```python
from build123d import *

# Parameters (mm, degrees)
SKETCH_1_R          = 3.4
EXTRUDE_1_DEPTH     = 11
SKETCH_2_R          = 3.4
EXTRUDE_2_DEPTH     = 3
SKETCH_3_R          = 3.4
CUT_EXTRUDE_1_DEPTH = 28.083205128
CUT_EXTRUDE_START   = -5
SKETCH_4_R          = 6
SKETCH_4_R_2        = 3.4
CUT_EXTRUDE_2_DEPTH = 5
CUT_EXTRUDE_3_DEPTH = 28.083205128
CUT_EXTRUDE_5_DEPTH = 28.083205128
SKETCH_8_R          = 3.4
EXTRUDE_3_DEPTH     = 1
CUT_EXTRUDE_START_2 = -1
CUT_EXTRUDE_6_DEPTH = 1
CUT_EXTRUDE_7_DEPTH = 1
CUT_EXTRUDE_START_3 = -10
CUT_EXTRUDE_8_DEPTH = 10
EXTRUDE_START       = -4
SKETCH_12_R         = 6
SKETCH_12_R_2       = 3.25
EXTRUDE_5_DEPTH     = 4


with BuildPart() as part:
    # 草图1 → 凸台-拉伸1 (new body)
    with BuildSketch(Plane.XY):
        with BuildLine():
            Line((-9.5, -17.5), (9.5, -17.5))
            ThreePointArc((9.5, -17.5), (15.156854249, -15.156854249), (17.5, -9.5))
            Line((17.5, -9.5), (17.5, 9.5))
            ThreePointArc((17.5, 9.5), (15.156854249, 15.156854249), (9.5, 17.5))
            Line((9.5, 17.5), (-9.5, 17.5))
            ThreePointArc((-9.5, 17.5), (-15.156854249, 15.156854249), (-17.5, 9.5))
            Line((-17.5, 9.5), (-17.5, -9.5))
            ThreePointArc((-17.5, -9.5), (-15.156854249, -15.156854249), (-9.5, -17.5))
        make_face()
        with Locations((10.606601718, 10.606601718)):
            Circle(SKETCH_1_R, mode=Mode.SUBTRACT)
        with Locations((10.606601718, -10.606601718)):
            Circle(SKETCH_1_R, mode=Mode.SUBTRACT)
        with Locations((-10.606601718, -10.606601718)):
            Circle(SKETCH_1_R, mode=Mode.SUBTRACT)
        with Locations((-10.606601718, 10.606601718)):
            Circle(SKETCH_1_R, mode=Mode.SUBTRACT)
    extrude(amount=EXTRUDE_1_DEPTH)

    # 草图2 → 凸台-拉伸2 (add)
    with BuildSketch(Plane(origin=(0, 0, 0), x_dir=(-1, 0, 0), z_dir=(0, 0, -1))):
        with Locations((10.606601718, -10.606601718)):
            Circle(SKETCH_2_R)
        with Locations((-10.606601718, -10.606601718)):
            Circle(SKETCH_2_R)
        with Locations((10.606601718, 10.606601718)):
            Circle(SKETCH_2_R)
        with Locations((-10.606601718, 10.606601718)):
            Circle(SKETCH_2_R)
    extrude(amount=-EXTRUDE_2_DEPTH)

    # 草图3 → 切除-拉伸1 (cut, through all)
    with BuildSketch(Plane.XY.offset(11)):
        Circle(SKETCH_3_R)
    extrude(amount=-CUT_EXTRUDE_1_DEPTH, mode=Mode.SUBTRACT)

    # 草图4 → 切除-拉伸2 (cut)
    with BuildSketch(Plane(origin=(0, 0, 0), x_dir=(-1, 0, 0), z_dir=(0, 0, -1)).offset(CUT_EXTRUDE_START)):
        Circle(SKETCH_4_R)
        with Locations(Location((0, 0, 0), (0, 0, 180))):
            Circle(SKETCH_4_R_2, mode=Mode.SUBTRACT)
    extrude(amount=CUT_EXTRUDE_2_DEPTH, mode=Mode.SUBTRACT)

    # 草图6 → 切除-拉伸3 (cut, through all)
    with BuildSketch(Plane(origin=(0, 0, 0), x_dir=(-1, 0, 0), z_dir=(0, 0, -1))):
        with BuildLine():
            Line((9.5, 17.5), (0, 17.5))
            Line((0, 17.5), (17.5, 0))
            Line((17.5, 0), (17.5, 9.5))
            ThreePointArc((17.5, 9.5), (15.156854249, 15.156854249), (9.5, 17.5))
        make_face()
        with BuildLine():
            Line((17.5, -9.5), (17.5, 0))
            Line((17.5, 0), (0, -17.5))
            Line((0, -17.5), (9.5, -17.5))
            ThreePointArc((9.5, -17.5), (15.156854249, -15.156854249), (17.5, -9.5))
        make_face()
    extrude(amount=-CUT_EXTRUDE_3_DEPTH, mode=Mode.SUBTRACT)

    # 草图7 → 切除-拉伸5 (cut, through all)
    with BuildSketch(Plane.XY.offset(11)):
        with BuildLine():
            Line((-7.222574041, -10.277425959), (0, -17.5))
            ThreePointArc((0, -17.5), (-7.248737342, 0), (0, 17.5))
            Line((0, 17.5), (-7.222574041, 10.277425959))
            ThreePointArc((-7.222574041, 10.277425959), (-8.202438662, 8.202438662), (-10.277425959, 7.222574041))
            Line((-10.277425959, 7.222574041), (-17.5, 0))
            Line((-17.5, 0), (-10.277425959, -7.222574041))
            ThreePointArc((-10.277425959, -7.222574041), (-8.202438662, -8.202438662), (-7.222574041, -10.277425959))
        make_face()
        with BuildLine():
            Line((-10.277425959, -7.222574041), (-7.222574041, -10.277425959))
            ThreePointArc((-7.222574041, -10.277425959), (-8.202438662, -8.202438662), (-10.277425959, -7.222574041))
        make_face()
        with BuildLine():
            ThreePointArc((-10.277425959, 7.222574041), (-8.202438662, 8.202438662), (-7.222574041, 10.277425959))
            Line((-7.222574041, 10.277425959), (-10.277425959, 7.222574041))
        make_face()
    extrude(amount=-CUT_EXTRUDE_5_DEPTH, mode=Mode.SUBTRACT)

    # 草图8 → 凸台-拉伸3 (add)
    with BuildSketch(Plane.XY.offset(11)):
        with BuildLine():
            Line((9.5, 17.5), (0, 17.5))
            ThreePointArc((0, 17.5), (-7.248737342, 0), (0, -17.5))
            Line((0, -17.5), (9.5, -17.5))
            ThreePointArc((9.5, -17.5), (15.156854249, -15.156854249), (17.5, -9.5))
            Line((17.5, -9.5), (17.5, 9.5))
            ThreePointArc((17.5, 9.5), (15.156854249, 15.156854249), (9.5, 17.5))
        make_face()
        Circle(SKETCH_8_R, mode=Mode.SUBTRACT)
        with Locations(Location((10.606601718, 10.606601718, 0), (0, 0, 180))):
            Circle(SKETCH_8_R, mode=Mode.SUBTRACT)
        with Locations(Location((10.606601718, -10.606601718, 0), (0, 0, 180))):
            Circle(SKETCH_8_R, mode=Mode.SUBTRACT)
    extrude(amount=EXTRUDE_3_DEPTH)

    # 草图9 → 切除-拉伸6 (cut)
    with BuildSketch(Plane.XY.offset(12).offset(CUT_EXTRUDE_START_2)):
        with BuildLine():
            Line((9.5, 17.5), (0, 17.5))
            ThreePointArc((0, 17.5), (-7.248737342, 0), (0, -17.5))
            Line((0, -17.5), (9.5, -17.5))
            ThreePointArc((9.5, -17.5), (15.156854249, -15.156854249), (17.5, -9.5))
            Line((17.5, -9.5), (17.5, 9.5))
            ThreePointArc((17.5, 9.5), (15.156854249, 15.156854249), (9.5, 17.5))
        make_face()
    extrude(amount=CUT_EXTRUDE_6_DEPTH, mode=Mode.SUBTRACT)

    # 草图10 → 切除-拉伸7 (cut)
    with BuildSketch(Plane(origin=(0, 0, 0), x_dir=(-1, 0, 0), z_dir=(0, 0, -1))):
        with BuildLine():
            Line((0, 17.5), (-9.5, 17.5))
            ThreePointArc((-9.5, 17.5), (-15.156854249, 15.156854249), (-17.5, 9.5))
            Line((-17.5, 9.5), (-17.5, -9.5))
            ThreePointArc((-17.5, -9.5), (-15.156854249, -15.156854249), (-9.5, -17.5))
            Line((-9.5, -17.5), (0, -17.5))
            ThreePointArc((0, -17.5), (7.248737342, 0), (0, 17.5))
        make_face()
    extrude(amount=-CUT_EXTRUDE_7_DEPTH, mode=Mode.SUBTRACT)

    # 草图11 → 切除-拉伸8 (cut)
    with BuildSketch(Plane(origin=(0, 0, 1), x_dir=(-1, 0, 0), z_dir=(0, 0, -1)).offset(CUT_EXTRUDE_START_3)):
        with BuildLine():
            Line((0, 17.5), (-9.5, 17.5))
            Line((-9.5, 17.5), (4.674526852, 5.540125608))
            ThreePointArc((4.674526852, 5.540125608), (6.573758833, 3.054486512), (7.248737342, 0))
            ThreePointArc((7.248737342, 0), (5.364851885, 9.470931753), (0, 17.5))
        make_face()
        with BuildLine():
            ThreePointArc((0, -17.5), (5.364851885, -9.470931753), (7.248737342, 0))
            ThreePointArc((7.248737342, 0), (6.573758833, -3.054486512), (4.674526852, -5.540125608))
            Line((4.674526852, -5.540125608), (-9.5, -17.5))
            Line((-9.5, -17.5), (0, -17.5))
        make_face()
    extrude(amount=CUT_EXTRUDE_8_DEPTH, mode=Mode.SUBTRACT)

    # 草图12 → 凸台-拉伸5 (add)
    with BuildSketch(Plane(origin=(0, 0, 1), x_dir=(-1, 0, 0), z_dir=(0, 0, -1)).offset(EXTRUDE_START)):
        Circle(SKETCH_12_R)
        Circle(SKETCH_12_R_2, mode=Mode.SUBTRACT)
    extrude(amount=EXTRUDE_5_DEPTH)


solid = part.part
```
Work out the finished part from the listing and answer in its coordinate system (mm). A direction names the side the tool comes from. Coordinates: 2 decimals unless noted, no trailing zeros. Loops run counter-clockwise (first coordinate to the right, second up) from the corner with the lowest first, then second, coordinate; pieces in that order, holes last. Notation, with made-up numbers: (84.5, 8) -> (143.5, 8) arc R7 ccw to (143.5, 12) -> close; hole circle Ø3 at (18.25, 24). An arc over 180 degrees is marked (long way). Answer as CSV lines item,"result".
Q1. For a pull along Y with two mould halves and no side action, classify faces 3 (the face through (2.51, 11.6, 6.07)), 4 (the face through (12.434, 13.473, 6.944)), 5 (the face through (2.314, -11.436, 6.07)), 6 (the face through (17.5, 0, 6)) as +Y half, -Y half, draft (parallel to the pull), parting line (faces both ways), or undercut.
Findings:
face 3,"+Y half"
face 4,"undercut"
face 5,"-Y half"
face 6,"draft"
Q2. The part is cut by section B-B on z = 9. Write down the section's boundary in (x, y), and give its area (3 significant figures).
Findings:
outline,"(-4.67, -5.54) -> (9.5, -17.5) arc R8 ccw to (17.5, -9.5) -> (17.5, 9.5) arc R8 ccw to (9.5, 17.5) -> (-4.67, 5.54) arc R7.25 ccw to start; hole circle Ø6.8 at (0, 0); hole circle Ø6.8 at (10.61, -10.61); hole circle Ø6.8 at (10.61, 10.61)"
area,"490 mm²"
Q3. Find the intervals of material crossed by probe 1 along Y at (x, z) = (10.25, 6.25); probe 2 along Y at (x, z) = (-0.25, 10.75); probe 3 along Y at (x, z) = (2.5, 3.25), in increasing order.
Findings:
probe 1,"y = -17.46 to -13.99, -7.23 to 7.23, 13.99 to 17.46"
probe 2,"y = -9.27 to -3.39, 3.39 to 9.27"
probe 3,"y = -11.59 to -2.08, 2.08 to 11.59"
Q4. A tool of negligible diameter and unlimited length cuts with its end or side. For faces 1 (the face through (11, -11, 3)), 2 (the face through (15.219, 15.094, 5.93)), from which of +Z, -Z, +X, -X, +Y, -Y can it reach the whole face along a straight path? Write none if from no direction.
Findings:
face 1,"+Z"
face 2,"+Z, -Z, +X, +Y"
Q5. The part is cut by section D-D on x = 13. Write down the section's boundary in (y, z).
Findings:
outline,"(-16.69, 1) -> (16.69, 1) -> (16.69, 11) -> (13.02, 11) -> (13.02, 3) -> (8.19, 3) -> (8.19, 11) -> (-8.19, 11) -> (-8.19, 3) -> (-13.02, 3) -> (-13.02, 11) -> (-16.69, 11) -> close"
Q6. The part is cut by section A-A on x = 0. Write down the section's boundary in (y, z), and give its area (3 significant figures).
Findings:
outline,"(-9.48, 1) -> (-3.25, 1) -> (-3.25, 5) -> (-3.4, 5) -> (-3.4, 11) -> (-9.48, 11) -> close; (3.25, 1) -> (9.48, 1) -> (9.48, 11) -> (3.4, 11) -> (3.4, 5) -> (3.25, 5) -> close"
area,"123 mm²"
Q7. Each of these flat-tipped pins is pushed along its axis until it touches: pin 1 (4 mm diameter, centred on x = 6, z = 9, fed in from -Y); pin 2 (3.5 mm diameter, centred on x = 9.5, y = 10, fed in from +Z); pin 3 (1 mm diameter, centred on x = 0, z = 4.5, fed in from -Y). Where does it stop, or does it pass through?
Findings:
pin 1,"stops at y = -16.23"
pin 2,"stops at z = 3"
pin 3,"stops at y = -9.91"
Q8. The part is cut by section C-C on y = -8.5. Write down the section's boundary in (x, z), and give its area (3 significant figures).
Findings:
outline,"(-1.17, 1) -> (17.5, 1) -> (17.5, 11) -> (13.28, 11) -> (13.28, 3) -> (7.94, 3) -> (7.94, 11) -> (-1.17, 11) -> close"
area,"144 mm²"
